Geometry check sheet. Reference: drawing and pictorial views, mm from the part's lowest x, y, z. A direction names the side the tool comes from. Round coordinates to 2 decimals unless told otherwise and drop trailing zeros. Write each loop counter-clockwise with the first axis right and the second up, starting at its lowest first coordinate (ties: lowest second). Pieces come first, ordered by that corner, then holes. Notation, with made-up numbers: (72.25, 39.5) -> (112.25, 39.5) arc R20 ccw to (112.25, 75.5) -> close; hole circle Ø1 at (48.25, 39). An arc over 180 degrees is marked (long way). Write item = value, one per line.
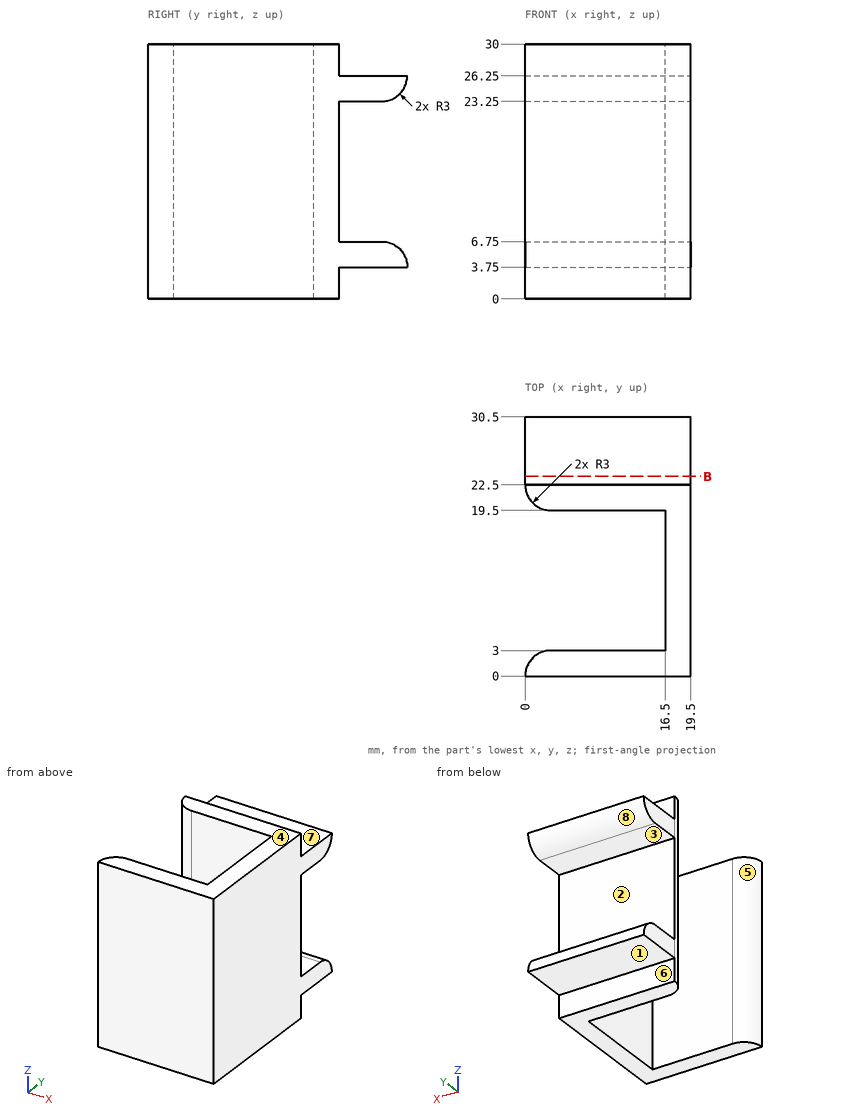
(1) Go/stop test with flat-tipped pins: P1, Ø1.9, axis at x = 11.5, z = 28.5, coming from the +Y side; P2, Ø4, axis at x = 11, y = 27, coming from the +Z side; P3, Ø18, axis at y = 11, z = 10.5, coming from the -X side. Record where each tip stops, or that it passes through.
Worked answers:
P1 = 22.5
P2 = 26.25
P3 = 0.76
(2) Material ranges on L1, parallel to Y at x = 13.75, z = 14.5; L2, parallel to Z at x = 2.25, y = 23.5; L3, parallel to X at y = 15, z = 21, recorded low to high. Write a range as [from, to].
Worked answers:
L1 = [0, 3], [19.5, 22.5]
L2 = [3.75, 6.75], [23.25, 26.25]
L3 = [16.5, 19.5]
(3) Access from +Z, -Z, +X, -X, +Y, -Y to the whole of each face (thin tool, end or side, straight path). Record for the marked faces 5, 6, 7 and 8.
Worked answers:
face_5 = +Z, -Z, -X
face_6 = -Z, +X, -X, +Y
face_7 = +Z, +X, -X, +Y
face_8 = +X, -X, +Y
(4) Sectioned sample at B-B on y = 23.5. Enter the section's corners in (x, z), then the cut area to 3 significant figures.
Worked answers:
outline = (0, 3.75) -> (19.5, 3.75) -> (19.5, 6.75) -> (0, 6.75) -> close; (0, 23.25) -> (19.5, 23.25) -> (19.5, 26.25) -> (0, 26.25) -> close
area = 117 mm²
(5) Release check for a two-part mould opening along Z. For the marked faces 1, 2, 3 and 4 record: pulls with the +Z half, pulls with the -Z half, needs draft (parallel to the pull), parting line crosses it, or undercut.
Worked answers:
face_1 = pulls with the -Z half
face_2 = undercut
face_3 = undercut
face_4 = pulls with the +Z half
